from build123d import *

# Parameters (mm, degrees)
SKETCH1_W                                       = 98
SKETCH1_H                                       = 80
BOSS_EXTRUDE1_DEPTH                             = 5
SKETCH2_W                                       = 7
SKETCH2_H                                       = 80
BOSS_EXTRUDE2_DEPTH                             = 8.5
SKETCH3_W                                       = 7
SKETCH3_H                                       = 80
BOSS_EXTRUDE3_DEPTH                             = 8.5
SKETCH8_W                                       = 84
SKETCH8_H                                       = 8.5
BOSS_EXTRUDE5_DEPTH                             = 5
SKETCH13_R                                      = 2.25
CUT_EXTRUDE7_DEPTH                              = 3.2
SKETCH15_R                                      = 1.5
CUT_EXTRUDE9_DEPTH                              = 3.2
SKETCH14_W                                      = 16
SKETCH14_H                                      = 16
CUT_EXTRUDE13_DEPTH                             = 3
SKETCH18_W                                      = 16
SKETCH18_H                                      = 12
CUT_EXTRUDE14_DEPTH                             = 64.822018144
SKETCH19_W                                      = 16
SKETCH19_H                                      = 5.672791846
CUT_EXTRUDE15_DEPTH                             = 3
SKETCH20_R                                      = 2.25
CUT_EXTRUDE20_DEPTH                             = 3.2
BOSS_EXTRUDE7_DEPTH                             = 10
BOSS_EXTRUDE9_DEPTH                             = 8
CSK_FOR_M3_FLAT_HEAD_MACHINE_SCREW1_D           = 3.4
CSK_FOR_M3_FLAT_HEAD_MACHINE_SCREW1_CSINK_D     = 6.3
CSK_FOR_M3_FLAT_HEAD_MACHINE_SCREW1_CSINK_ANGLE = 90
SKETCH51_R                                      = 17.75
CUT_EXTRUDE23_DEPTH                             = 8
CUT_EXTRUDE24_START                             = -8
SKETCH52_R                                      = 17.75
CUT_EXTRUDE24_DEPTH                             = 8
SKETCH42_R                                      = 2.25
CUT_EXTRUDE25_DEPTH                             = 4.25
SKETCH53_R                                      = 2.25
CUT_EXTRUDE26_DEPTH                             = 8.25
SKETCH54_R                                      = 1.5
CUT_EXTRUDE27_DEPTH                             = 13.25
CUT_EXTRUDE28_DEPTH                             = 5
CUT_EXTRUDE29_START                             = -13.25
SKETCH56_R                                      = 1.5
CUT_EXTRUDE29_DEPTH                             = 13.25
CUT_EXTRUDE30_START                             = -5
CUT_EXTRUDE30_DEPTH                             = 5
SKETCH65_W                                      = 20
SKETCH65_H                                      = 14.4
CUT_EXTRUDE31_DEPTH                             = 77.401897882
CUT_EXTRUDE33_DEPTH                             = 13.5
SKETCH75_W                                      = 28.5
SKETCH75_H                                      = 7
CUT_EXTRUDE39_DEPTH                             = 11
SKETCH80_W                                      = 5
SKETCH80_H                                      = 12
CUT_EXTRUDE42_DEPTH                             = 77.401897882
SKETCH82_W                                      = 0.8
SKETCH82_H                                      = 7
SKETCH82_W_2                                    = 0.2
CUT_EXTRUDE43_DEPTH                             = 11
SKETCH84_W                                      = 5.5
SKETCH84_H                                      = 8.5
SKETCH84_R                                      = 1.5
BOSS_EXTRUDE10_DEPTH                            = 3.5
SKETCH86_W                                      = 5.5
SKETCH86_H                                      = 3.5
BOSS_EXTRUDE11_DEPTH                            = 3.5


with BuildPart() as part:
    # Sketch1 → Boss-Extrude1 (new body)
    with BuildSketch(Plane.XY):
        Rectangle(SKETCH1_W, SKETCH1_H)
    extrude(amount=BOSS_EXTRUDE1_DEPTH)

    # Sketch2 → Boss-Extrude2 (add)
    with BuildSketch(Plane.XY.offset(5)):
        with Locations((-45.5, 0)):
            Rectangle(SKETCH2_W, SKETCH2_H)
    extrude(amount=BOSS_EXTRUDE2_DEPTH)

    # Sketch3 → Boss-Extrude3 (add)
    with BuildSketch(Plane.XY.offset(5)):
        with Locations((45.5, 0)):
            Rectangle(SKETCH3_W, SKETCH3_H)
    extrude(amount=BOSS_EXTRUDE3_DEPTH)

    # Sketch8 → Boss-Extrude5 (add)
    with BuildSketch(Plane(origin=(0, 40, 0), x_dir=(1, 0, 0), z_dir=(0, 1, 0))):
        with Locations((0, -9.25)):
            Rectangle(SKETCH8_W, SKETCH8_H)
    extrude(amount=-BOSS_EXTRUDE5_DEPTH)

    # Sketch13 → Cut-Extrude7 (cut)
    with BuildSketch(Plane.XY.offset(5)):
        with Locations((0, -10)):
            Circle(SKETCH13_R)
    extrude(amount=-CUT_EXTRUDE7_DEPTH, mode=Mode.SUBTRACT)

    # Sketch15 → Cut-Extrude9 (cut)
    with BuildSketch(Plane.XY.offset(5)):
        with Locations((-37.62, 17)):
            Circle(SKETCH15_R)
        with Locations((-20.38, 17)):
            Circle(SKETCH15_R)
        with Locations((-37.62, -25)):
            Circle(SKETCH15_R)
        with Locations((-20.38, -25)):
            Circle(SKETCH15_R)
        with Locations((20.38, -25)):
            Circle(SKETCH15_R)
        with Locations((37.62, -25)):
            Circle(SKETCH15_R)
        with Locations((37.62, 17)):
            Circle(SKETCH15_R)
        with Locations((20.38, 17)):
            Circle(SKETCH15_R)
    extrude(amount=-CUT_EXTRUDE9_DEPTH, mode=Mode.SUBTRACT)

    # Sketch14 → Cut-Extrude13 (cut)
    with BuildSketch(Plane.XY.offset(5)):
        with Locations((0, 6.327208154)):
            Rectangle(SKETCH14_W, SKETCH14_H)
    extrude(amount=-CUT_EXTRUDE13_DEPTH, mode=Mode.SUBTRACT)

    # Sketch18 → Cut-Extrude14 (cut, through all)
    with BuildSketch(Plane.XY.offset(5)):
        with Locations((0, 26)):
            Rectangle(SKETCH18_W, SKETCH18_H)
    extrude(amount=-CUT_EXTRUDE14_DEPTH, mode=Mode.SUBTRACT)

    # Sketch19 → Cut-Extrude15 (cut)
    with BuildSketch(Plane.XY.offset(5)):
        with Locations((0, 17.163604077)):
            Rectangle(SKETCH19_W, SKETCH19_H)
    extrude(amount=-CUT_EXTRUDE15_DEPTH, mode=Mode.SUBTRACT)

    # Sketch20 → Cut-Extrude20 (cut)
    with BuildSketch(Plane(origin=(0, 0, 0), x_dir=(-1, 0, 0), z_dir=(0, 0, -1))):
        with Locations((18.25, 21.5)):
            Circle(SKETCH20_R)
        with Locations((-18.25, 21.5)):
            Circle(SKETCH20_R)
        with Locations((18.25, -15)):
            Circle(SKETCH20_R)
        with Locations((-18.25, -15)):
            Circle(SKETCH20_R)
    extrude(amount=-CUT_EXTRUDE20_DEPTH, mode=Mode.SUBTRACT)

    # Sketch26 → Boss-Extrude7 (add)
    with BuildSketch(Plane(origin=(0, -40, 0), x_dir=(-1, 0, 0), z_dir=(0, -1, 0))):
        Polygon((49, -13.5), (42, -13.5), (42, -5), (-42, -5), (-42, -13.5), (-49, -13.5), (-49, 0), (49, 0), align=None)
    extrude(amount=BOSS_EXTRUDE7_DEPTH)

    # Sketch47 → Boss-Extrude9 (add)
    with BuildSketch(Plane(origin=(0, -50, 0), x_dir=(-1, 0, 0), z_dir=(0, -1, 0))):
        Polygon((49, -13.5), (42, -13.5), (42, -5), (-42, -5), (-42, -13.5), (-49, -13.5), (-49, 0), (49, 0), align=None)
    extrude(amount=BOSS_EXTRUDE9_DEPTH)

    # CSK for M3 Flat Head Machine Screw1 (through all)
    with Locations(Plane.XY.offset(5)):
        with Locations((28, -30.88), (0, -30.88), (-28, -30.88)):
            CounterSinkHole(CSK_FOR_M3_FLAT_HEAD_MACHINE_SCREW1_D / 2, CSK_FOR_M3_FLAT_HEAD_MACHINE_SCREW1_CSINK_D / 2, counter_sink_angle=CSK_FOR_M3_FLAT_HEAD_MACHINE_SCREW1_CSINK_ANGLE)

    # Sketch51 → Cut-Extrude23 (cut)
    with BuildSketch(Plane.ZY.offset(49)):
        with Locations((-13, -44)):
            Circle(SKETCH51_R)
    extrude(amount=-CUT_EXTRUDE23_DEPTH, mode=Mode.SUBTRACT)

    # Sketch52 → Cut-Extrude24 (cut)
    with BuildSketch(Plane(origin=(49, 0, 0), x_dir=(0, 0, -1), z_dir=(1, 0, 0)).offset(CUT_EXTRUDE24_START)):
        with Locations((13, -44)):
            Circle(SKETCH52_R)
    extrude(amount=CUT_EXTRUDE24_DEPTH, mode=Mode.SUBTRACT)

    # Sketch42 → Cut-Extrude25 (cut)
    with BuildSketch(Plane.XY.offset(13.5)):
        with Locations((-45.5, 36.5)):
            Circle(SKETCH42_R)
        with Locations((45.5, 36.5)):
            Circle(SKETCH42_R)
    extrude(amount=-CUT_EXTRUDE25_DEPTH, mode=Mode.SUBTRACT)

    # Sketch53 → Cut-Extrude26 (cut)
    with BuildSketch(Plane.XY.offset(13.5)):
        with Locations((-45.5, -25.5)):
            Circle(SKETCH53_R)
        with Locations((45.5, -25.5)):
            Circle(SKETCH53_R)
    extrude(amount=-CUT_EXTRUDE26_DEPTH, mode=Mode.SUBTRACT)

    # Sketch54 → Cut-Extrude27 (cut)
    with BuildSketch(Plane.ZY.offset(49)):
        with Locations((3, 37)):
            Circle(SKETCH54_R)
    extrude(amount=-CUT_EXTRUDE27_DEPTH, mode=Mode.SUBTRACT)

    # Sketch55 → Cut-Extrude28 (cut)
    with BuildSketch(Plane.ZY.offset(49)):
        with BuildLine():
            Line((5.5, 37), (5.5, 40))
            Line((5.5, 40), (0, 40))
            Line((0, 40), (0, 34.5))
            Line((0, 34.5), (3, 34.5))
            ThreePointArc((3, 34.5), (4.767766953, 35.232233047), (5.5, 37))
        make_face()
    extrude(amount=-CUT_EXTRUDE28_DEPTH, mode=Mode.SUBTRACT)

    # Sketch56 → Cut-Extrude29 (cut)
    with BuildSketch(Plane(origin=(49, 0, 0), x_dir=(0, 0, -1), z_dir=(1, 0, 0)).offset(CUT_EXTRUDE29_START)):
        with Locations(Location((-3, 37, 0), (0, 0, 180))):
            Circle(SKETCH56_R)
    extrude(amount=CUT_EXTRUDE29_DEPTH, mode=Mode.SUBTRACT)

    # Sketch57 → Cut-Extrude30 (cut)
    with BuildSketch(Plane(origin=(49, 0, 0), x_dir=(0, 0, -1), z_dir=(1, 0, 0)).offset(CUT_EXTRUDE30_START)):
        with BuildLine():
            Line((-5.5, 37), (-5.5, 40))
            Line((-5.5, 40), (0, 40))
            Line((0, 40), (0, 34.5))
            Line((0, 34.5), (-3, 34.5))
            ThreePointArc((-3, 34.5), (-4.767766953, 35.232233047), (-5.5, 37))
        make_face()
    extrude(amount=CUT_EXTRUDE30_DEPTH, mode=Mode.SUBTRACT)

    # Sketch65 → Cut-Extrude31 (cut, through all)
    with BuildSketch(Plane.XY.offset(5)):
        with Locations((32, -4)):
            Rectangle(SKETCH65_W, SKETCH65_H)
        with Locations((-32, -4)):
            Rectangle(SKETCH65_W, SKETCH65_H)
    extrude(amount=-CUT_EXTRUDE31_DEPTH, mode=Mode.SUBTRACT)

    # Sketch69 → Cut-Extrude33 (cut)
    with BuildSketch(Plane.XZ.offset(-35)):
        Polygon((0, 12.45), (3.2, 12.45), (3.2, 6.05), (-3.2, 6.05), (-3.2, 12.45), align=None)
    extrude(amount=-CUT_EXTRUDE33_DEPTH, mode=Mode.SUBTRACT)

    # Sketch75 → Cut-Extrude39 (cut)
    with BuildSketch(Plane.XY.offset(13.5)):
        with Locations((-4.95, 35)):
            Rectangle(SKETCH75_W, SKETCH75_H)
    extrude(amount=-CUT_EXTRUDE39_DEPTH, mode=Mode.SUBTRACT)

    # Sketch80 → Cut-Extrude42 (cut, through all)
    with BuildSketch(Plane.XY.offset(5)):
        with Locations((-10.5, 26)):
            Rectangle(SKETCH80_W, SKETCH80_H)
    extrude(amount=-CUT_EXTRUDE42_DEPTH, mode=Mode.SUBTRACT)

    # Sketch82 → Cut-Extrude43 (cut)
    with BuildSketch(Plane.XY.offset(13.5)):
        with Locations((-19.6, 35)):
            Rectangle(SKETCH82_W, SKETCH82_H)
        with Locations((9.4, 35)):
            Rectangle(SKETCH82_W_2, SKETCH82_H)
    extrude(amount=-CUT_EXTRUDE43_DEPTH, mode=Mode.SUBTRACT)

    # Sketch84 → Boss-Extrude10 (add)
    # profile 1 of 2: a face of its own
    with BuildSketch(Plane.XZ.offset(-38.5)):
        with Locations((-17.25, 9.25)):
            Rectangle(SKETCH84_W, SKETCH84_H)
        with Locations(Location((-17, 9.05, 0), (0, 0, 270))):
            Circle(SKETCH84_R, mode=Mode.SUBTRACT)
    # profile 2 of 2: a face of its own
    with BuildSketch(Plane.XZ.offset(-38.5)):
        with Locations((6.75, 9.25)):
            Rectangle(SKETCH84_W, SKETCH84_H)
        with Locations(Location((6.5, 9.05, 0), (0, 0, 270))):
            Circle(SKETCH84_R, mode=Mode.SUBTRACT)
    extrude(amount=BOSS_EXTRUDE10_DEPTH)

    # Sketch86 → Boss-Extrude11 (add)
    with BuildSketch(Plane.XY.offset(2.5)):
        with Locations((-17.25, 36.75)):
            Rectangle(SKETCH86_W, SKETCH86_H)
        with Locations((6.75, 36.75)):
            Rectangle(SKETCH86_W, SKETCH86_H)
    extrude(amount=BOSS_EXTRUDE11_DEPTH)


solid = part.part
Verification items for the finished model (mm, model axes). A direction names the side the tool comes from. Coordinates: 2 decimals unless noted, no trailing zeros. Write each loop counter-clockwise with the first axis right and the second up, starting at its lowest first coordinate (ties: lowest second). Pieces come first, ordered by that corner, then holes. Notation, with made-up numbers: (8, 43) -> (50, 43) arc R19 cw to (50, 77) -> close; hole circle Ø10 at (22, -9). An arc over 180 degrees is marked (long way). One line per item, written item: value. Start each with the question number.
Q1. Go/stop test with flat-tipped pins: P1, Ø2.5, axis at x = 18.25, y = 21.5, coming from the +Z side; P2, Ø2, axis at x = -5, y = 20.5, coming from the +Z side. Record where each tip stops, or that it passes through.
Q2. Access from +Z, -Z, +X, -X, +Y, -Y to the whole of each face (thin tool, end or side, straight path). Record for faces 4 (the flat face through (-18, 22, 3.2)), 5 (the flat face through (20, -25, 1.8)), 6 (the flat face through (-3, 32, 1)).
Q3. Cross-section at A-A on x = 28. Enter the section's corners in (y, z), and give its area (3 significant figures).
Q4. Thickness scan on L1, parallel to X at y = 36.7, z = 9.05; L2, parallel to X at y = -44, z = 10; L3, parallel to Y at x = 18.25, z = 2.35. Record the ranges inside material, lowest first. Write a range as from..to.
Q5. Cross-section at C-C on x = -6. Enter the section's corners in (y, z), and give its area (3 significant figures).
Q6. Cross-section at D-D on x = 45.5. Enter the section's corners in (y, z), and give its area (3 significant figures).
Q7. Mould release check, pull along Z, two halves, no side actions. Record for faces 1 (the cylindrical face through (-15.735, 36.774, 8.244)), 2 (the flat face through (-28, 35, 9)), 3 (the flat face through (-20, -25, 1.8)): pulls with the +Z half, pulls with the -Z half, needs draft (parallel to the pull), parting line crosses it, or undercut.
Q8. Cross-section at B-B on y = -3. Enter the section's corners in (x, z).
Checked values:
1. P1: stops at z = 5
1. P2: stops at z = 2
2. face 4: -Z
2. face 5: +Z
2. face 6: +Z, -Z
3. outline: (-58, 0) -> (-32.58, 0) -> (-32.58, 3.55) -> (-34.03, 5) -> (-58, 5) -> close; (-29.18, 0) -> (-11.2, 0) -> (-11.2, 5) -> (-27.73, 5) -> (-29.18, 3.55) -> close; (3.2, 0) -> (40, 0) -> (40, 13.5) -> (35, 13.5) -> (35, 5) -> (3.2, 5) -> close
3. area: 441 mm²
4. L1: x = -49..-18.5, -15.5..-14.5, 4..5, 8..49
4. L2: x = -49..-42, 42..49
4. L3: y = -58..-17.25, -12.75..19.25, 23.75..40
5. outline: (-58, 0) -> (20, 0) -> (20, 2) -> (-1.67, 2) -> (-1.67, 5) -> (-58, 5) -> close; (32, 0) -> (40, 0) -> (40, 13.5) -> (38.5, 13.5) -> (38.5, 2.5) -> (32, 2.5) -> close
5. area: 361 mm²
6. outline: (-58, 0) -> (-56.09, 0) arc R17.75 cw to (-31.91, 0) -> (34.5, 0) -> (34.5, 3) arc R2.5 cw to (37, 5.5) -> (40, 5.5) -> (40, 13.5) -> (38.75, 13.5) -> (38.75, 9.25) -> (34.25, 9.25) -> (34.25, 13.5) -> (-23.25, 13.5) -> (-23.25, 5.25) -> (-27.75, 5.25) -> (-27.75, 13.5) -> (-58, 13.5) -> close
6. area: 1,160 mm²
7. face 1: undercut
7. face 2: needs draft
7. face 3: pulls with the +Z half
8. outline: (-49, 0) -> (-42, 0) -> (-42, 13.5) -> (-49, 13.5) -> close; (-22, 0) -> (22, 0) -> (22, 5) -> (-22, 5) -> close; (42, 0) -> (49, 0) -> (49, 13.5) -> (42, 13.5) -> close
